```python
from build123d import *

# Parameters (mm, degrees)
SKETCH1_R           = 2.15
SKETCH1_R_2         = 2.1
BOSS_EXTRUDE1_DEPTH = 6.35
SKETCH2_R           = 2.1
CUT_EXTRUDE1_DEPTH  = 5


with BuildPart() as part:
    # Sketch1 → Boss-Extrude1 (new body)
    with BuildSketch(Plane.XY):
        Polygon((-14.5, 164.786291501), (-29.2, 184.786291501), (-70.5, 184.786291501), (-70.5, 152.786291501), (-49.5, 131.786291501), (-49.5, -112.803421473), (-90, -135.112557197), (-90, -216.825), (-110, -216.825), (-110, -221.825), (-90, -241.825), (-90, -345.112557197), (0, -345.112557197), (0, -240.441757757), (-57.914505889, -240.441757757), (-57.914505889, -179.526253392), (-14.5, -153.791774149), align=None)
        with Locations((-19.5, 157.286291501)):
            Circle(SKETCH1_R, mode=Mode.SUBTRACT)
        with Locations((-42.5, 157.286291501)):
            Circle(SKETCH1_R, mode=Mode.SUBTRACT)
        with Locations((-65.5, 157.286291501)):
            Circle(SKETCH1_R, mode=Mode.SUBTRACT)
        with Locations((-84, -213.65)):
            Circle(SKETCH1_R_2, mode=Mode.SUBTRACT)
        with Locations((-63.914505889, -213.65)):
            Circle(SKETCH1_R_2, mode=Mode.SUBTRACT)
        with BuildLine():
            Line((-42.5, 181.936291501), (-32.5, 181.936291501))
            ThreePointArc((-32.5, 181.936291501), (-30.35, 179.786291501), (-32.5, 177.636291501))
            Line((-32.5, 177.636291501), (-42.5, 177.636291501))
            ThreePointArc((-42.5, 177.636291501), (-44.65, 179.786291501), (-42.5, 181.936291501))
        make_face(mode=Mode.SUBTRACT)
        with BuildLine():
            Line((-57.5, 181.936291501), (-47.5, 181.936291501))
            ThreePointArc((-47.5, 181.936291501), (-45.35, 179.786291501), (-47.5, 177.636291501))
            Line((-47.5, 177.636291501), (-57.5, 177.636291501))
            ThreePointArc((-57.5, 177.636291501), (-59.65, 179.786291501), (-57.5, 181.936291501))
        make_face(mode=Mode.SUBTRACT)
        with BuildLine():
            Line((-37.5, 171.936291501), (-27.5, 171.936291501))
            ThreePointArc((-27.5, 171.936291501), (-25.35, 169.786291501), (-27.5, 167.636291501))
            Line((-27.5, 167.636291501), (-37.5, 167.636291501))
            ThreePointArc((-37.5, 167.636291501), (-39.65, 169.786291501), (-37.5, 171.936291501))
        make_face(mode=Mode.SUBTRACT)
    extrude(amount=BOSS_EXTRUDE1_DEPTH)

    # Sketch2 → Cut-Extrude1 (cut)
    with BuildSketch(Plane(origin=(0, -216.825, 0), x_dir=(-1, 0, 0), z_dir=(0, 1, 0))):
        with Locations((95.5, 3.175)):
            Circle(SKETCH2_R)
        with Locations((104.5, 3.175)):
            Circle(SKETCH2_R)
    extrude(amount=-CUT_EXTRUDE1_DEPTH, mode=Mode.SUBTRACT)


solid = part.part
```
Verification items for the finished model (mm, model axes). A direction names the side the tool comes from. Coordinates: 2 decimals unless noted, no trailing zeros. Loops run counter-clockwise (first coordinate to the right, second up) from the corner with the lowest first, then second, coordinate; pieces in that order, holes last. Notation, with made-up numbers: (52.25, 34.25) - (101.25, 34.25) arc R25 cw to (101.25, 71.25) - close; hole circle Ø2 at (3.25, 5). An arc over 180 degrees is marked (long way). Return JSON: item names as keys, results as strings.
1. Thickness scan on L1, parallel to X at y = 157.5, z = 5.25; L2, parallel to Z at x = -95, y = -218; L3, parallel to Y at x = -65, z = 4.25. Record the ranges inside material, lowest first.
Established:
{"L1": "x = -70.5 to -67.64, -63.36 to -44.64, -40.36 to -21.64, -17.36 to -14.5", "L2": "z = 0 to 1.14, 5.21 to 6.35", "L3": "y = -345.11 to -215.45, -211.85 to -121.34, 147.29 to 155.2, 159.38 to 184.79"}
2. Section check A-A, the plane y = -32.5. Record the boundary of the cut face in (x, z).
Established:
{"outline": "(-49.5, 0) - (-14.5, 0) - (-14.5, 6.35) - (-49.5, 6.35) - close"}
3. Go/stop test with flat-tipped pins: pin 1 (3 mm diameter, centred on x = -23, z = 2, fed in from +Y); pin 2 (1.5 mm diameter, centred on x = -83, z = 1.5, fed in from +Y); pin 3 (3 mm diameter, centred on x = -105, z = 2, fed in from +Y) (3 decimals); pin 4 (3.5 mm diameter, centred on x = -84, y = -213.65, fed in from -Z). Record where each tip stops, or that it passes through.
Established:
{"pin 1": "stops at y = 178.39", "pin 2": "stops at y = -130.84", "pin 3": "stops at y = -216.825", "pin 4": "passes through"}
4. Tool access check on faces 1 (the flat face through (-60.147, 142.433, 3.131)), 2 (the flat face through (-21.75, 174.65, 3.13)). Record the directions out of +Z, -Z, +X, -X, +Y, -Y that give a thin tool (end or side, any length) a straight path to the whole face; none if there is none.
Established:
{"face 1": "+Z, -Z, -X", "face 2": "+Z, -Z, +X, +Y"}
5. Mould release check, pull along Y, two halves, no side actions. Record for faces 3 (the flat face through (-69.466, -123.802, 3.131)), 4 (the flat face through (-36.51, -166.84, 3.13)), 5 (the flat face through (-44, -135, 6.35)), 6 (the flat face through (-100.14, -231.685, 3.131)): +Y half, -Y half, draft (parallel to the pull), parting line (faces both ways), or undercut.
Established:
{"face 3": "undercut", "face 4": "undercut", "face 5": "draft", "face 6": "-Y half"}
